```python
from build123d import *

# Parameters (mm, degrees)
SKETCH_2_R               = 2.55
EXTRUDE_1_DEPTH          = 310
CUT_EXTRUDE_1_DEPTH      = 311.805405358
CUT_EXTRUDE_1_DEPTH_BACK = 311.805405358
SKETCH_3_R               = 3


with BuildPart() as part:
    # 草图2 → 凸台-拉伸1 (new body)
    with BuildSketch(Plane.XY):
        with BuildLine():
            Line((-3.9, 2.839339828), (-6.560660172, 5.5))
            Line((-6.560660172, 5.5), (-8.2, 5.5))
            Line((-8.2, 5.5), (-8.2, 3.1))
            Line((-8.2, 3.1), (-9.45, 3.1))
            Line((-9.45, 3.1), (-9.45, 3.65))
            Line((-9.45, 3.65), (-10, 3.65))
            Line((-10, 3.65), (-10, 8.5))
            ThreePointArc((-10, 8.5), (-9.560660172, 9.560660172), (-8.5, 10))
            Line((-8.5, 10), (-3.65, 10))
            Line((-3.65, 10), (-3.65, 9.45))
            Line((-3.65, 9.45), (-3.1, 9.45))
            Line((-3.1, 9.45), (-3.1, 8.2))
            Line((-3.1, 8.2), (-5.5, 8.2))
            Line((-5.5, 8.2), (-5.5, 6.560660172))
            Line((-5.5, 6.560660172), (-2.839339828, 3.9))
            Line((-2.839339828, 3.9), (2.839339828, 3.9))
            Line((2.839339828, 3.9), (5.5, 6.560660172))
            Line((5.5, 6.560660172), (5.5, 8.2))
            Line((5.5, 8.2), (3.1, 8.2))
            Line((3.1, 8.2), (3.1, 9.45))
            Line((3.1, 9.45), (3.65, 9.45))
            Line((3.65, 9.45), (3.65, 10))
            Line((3.65, 10), (8.5, 10))
            ThreePointArc((8.5, 10), (9.560660172, 9.560660172), (10, 8.5))
            Line((10, 8.5), (10, 3.65))
            Line((10, 3.65), (9.45, 3.65))
            Line((9.45, 3.65), (9.45, 3.1))
            Line((9.45, 3.1), (8.2, 3.1))
            Line((8.2, 3.1), (8.2, 5.5))
            Line((8.2, 5.5), (6.560660172, 5.5))
            Line((6.560660172, 5.5), (3.9, 2.839339828))
            Line((3.9, 2.839339828), (3.9, -2.839339828))
            Line((3.9, -2.839339828), (6.560660172, -5.5))
            Line((6.560660172, -5.5), (8.2, -5.5))
            Line((8.2, -5.5), (8.2, -3.1))
            Line((8.2, -3.1), (9.45, -3.1))
            Line((9.45, -3.1), (9.45, -3.65))
            Line((9.45, -3.65), (10, -3.65))
            Line((10, -3.65), (10, -8.5))
            ThreePointArc((10, -8.5), (9.560660172, -9.560660172), (8.5, -10))
            Line((8.5, -10), (3.65, -10))
            Line((3.65, -10), (3.65, -9.45))
            Line((3.65, -9.45), (3.1, -9.45))
            Line((3.1, -9.45), (3.1, -8.2))
            Line((3.1, -8.2), (5.5, -8.2))
            Line((5.5, -8.2), (5.5, -6.560660172))
            Line((5.5, -6.560660172), (2.839339828, -3.9))
            Line((2.839339828, -3.9), (-2.839339828, -3.9))
            Line((-2.839339828, -3.9), (-5.5, -6.560660172))
            Line((-5.5, -6.560660172), (-5.5, -8.2))
            Line((-5.5, -8.2), (-3.1, -8.2))
            Line((-3.1, -8.2), (-3.1, -9.45))
            Line((-3.1, -9.45), (-3.65, -9.45))
            Line((-3.65, -9.45), (-3.65, -10))
            Line((-3.65, -10), (-8.5, -10))
            ThreePointArc((-8.5, -10), (-9.560660172, -9.560660172), (-10, -8.5))
            Line((-10, -8.5), (-10, -3.65))
            Line((-10, -3.65), (-9.45, -3.65))
            Line((-9.45, -3.65), (-9.45, -3.1))
            Line((-9.45, -3.1), (-8.2, -3.1))
            Line((-8.2, -3.1), (-8.2, -5.5))
            Line((-8.2, -5.5), (-6.560660172, -5.5))
            Line((-6.560660172, -5.5), (-3.9, -2.839339828))
            Line((-3.9, -2.839339828), (-3.9, 2.839339828))
        make_face()
        Circle(SKETCH_2_R, mode=Mode.SUBTRACT)
    extrude(amount=EXTRUDE_1_DEPTH)

    # 草图3 → 切除-拉伸1 (cut, two sides: drawn at the far end of the back side and taken through both)
    with BuildSketch(Plane.XZ.offset(10).offset(-CUT_EXTRUDE_1_DEPTH_BACK)):
        with Locations(Location((0, 90, 0), (0, 0, 341.164003842))):
            Circle(SKETCH_3_R)
    extrude(amount=CUT_EXTRUDE_1_DEPTH + CUT_EXTRUDE_1_DEPTH_BACK, mode=Mode.SUBTRACT)


solid = part.part
```
Verification items for the finished model (mm, model axes). A direction names the side the tool comes from. Coordinates: 2 decimals unless noted, no trailing zeros. Loops run counter-clockwise (first coordinate to the right, second up) from the corner with the lowest first, then second, coordinate; pieces in that order, holes last. Notation, with made-up numbers: (53.25, 11) -> (85.25, 11) arc R29 cw to (85.25, 34) -> close; hole circle Ø2 at (-30.75, 77). An arc over 180 degrees is marked (long way). Answer in a Markdown table with one row per item. Add a question column.
1. Section check A-A, the plane y = 0. Enter the section's corners in (x, z), then the cut area to 3 significant figures.
2. Depth check by flat-ended pin: P1, Ø5, axis at x = -3.5, z = 207.5, coming from the +Y side; P2, Ø6, axis at x = 0, z = 77.5, coming from the +Y side; P3, Ø1, axis at x = -3, z = 253, coming from the -Y side; P4, Ø4.5, axis at x = 0.5, z = 165.5, coming from the -Y side. Enter the tip coordinate at first touch or a pass-through.
3. Access from +Z, -Z, +X, -X, +Y, -Y to the whole of each face (thin tool, end or side, straight path). Record for faces 1 (the face through (-3.9, 0, 153)), 2 (the face through (-10, -6, 153)), 3 (the face through (-6, -10, 153)), 4 (the face through (0, 3.9, 44)), 5 (the face through (0, -3.9, 44)).
4. Section check B-B, the plane x = 0. Enter the section's corners in (y, z), then the cut area to 3 significant figures.
5. Material ranges on probe 1 along Y at (x, z) = (-8, 44.5); probe 2 along X at (y, z) = (6.5, 216), recorded low to high. Write a range as [from, to].
6. Draft check along Z on faces 6 (the face through (-2.794, 0.057, 91.092)), 7 (the face through (2, 2, 0)), 8 (the face through (3.9, 0, 153)). Enter one of: +Z half, -Z half, draft (parallel to the pull), parting line (faces both ways), or undercut.
Derived:
| question | item | result |
|---|---|---|
| 1 | outline | (-3.9, 0) -> (-2.55, 0) -> (-2.55, 88.42) arc R3 cw to (-2.55, 91.58) -> (-2.55, 310) -> (-3.9, 310) -> close; (2.55, 0) -> (3.9, 0) -> (3.9, 310) -> (2.55, 310) -> (2.55, 91.58) arc R3 cw to (2.55, 88.42) -> close |
| 1 | area | 835 mm² |
| 2 | P1 | stops at y = 10 |
| 2 | P2 | stops at y = 4.06 |
| 2 | P3 | stops at y = -9.45 |
| 2 | P4 | stops at y = -3.9 |
| 3 | face 1 | +Z, -Z, -X |
| 3 | face 2 | +Z, -Z, -X, +Y, -Y |
| 3 | face 3 | +Z, -Z, +X, -X, -Y |
| 3 | face 4 | +Z, -Z, +Y |
| 3 | face 5 | +Z, -Z, -Y |
| 4 | outline | (-3.9, 0) -> (-2.55, 0) -> (-2.55, 87) -> (-3.9, 87) -> close; (-3.9, 93) -> (-2.55, 93) -> (-2.55, 310) -> (-3.9, 310) -> close; (2.55, 0) -> (3.9, 0) -> (3.9, 87) -> (2.55, 87) -> close; (2.55, 93) -> (3.9, 93) -> (3.9, 310) -> (2.55, 310) -> close |
| 4 | area | 821 mm² |
| 5 | probe 1 | y = [-10, -5.5], [5.5, 10] |
| 5 | probe 2 | x = [-10, -5.44], [5.44, 10] |
| 6 | face 6 | undercut |
| 6 | face 7 | -Z half |
| 6 | face 8 | draft |
